from build123d import *

# Parameters (mm, degrees)
SKETCH4_R           = 59
BOSS_EXTRUDE3_DEPTH = 2
SKETCH5_R           = 1.375
BOSS_EXTRUDE5_DEPTH = 7
SKETCH8_R           = 2.375
BOSS_EXTRUDE6_DEPTH = 2
BOSS_EXTRUDE7_DEPTH = 18
SKETCH10_R          = 7.5
CUT_EXTRUDE1_DEPTH  = 18
SKETCH12_R          = 57.5
CUT_EXTRUDE2_DEPTH  = 5
CUT_EXTRUDE3_DEPTH  = 5.5
SKETCH15_R          = 89.714021058
SKETCH15_R_2        = 57
CUT_EXTRUDE4_DEPTH  = 22
SKETCH16_R          = 62.462022857
CUT_EXTRUDE8_DEPTH  = 52
CUT_EXTRUDE9_DEPTH  = 52
SKETCH18_R          = 80.62246508
SKETCH18_R_2        = 55
CUT_EXTRUDE10_DEPTH = 10
SKETCH19_R          = 55
BOSS_EXTRUDE8_DEPTH = 2
SKETCH20_R          = 6.25
CUT_EXTRUDE11_DEPTH = 2
SKETCH21_W          = 10
SKETCH21_H          = 50
CUT_EXTRUDE12_DEPTH = 3
SKETCH22_R          = 40.394642533
CUT_EXTRUDE13_DEPTH = 10


with BuildPart() as part:
    # Sketch4 → Boss-Extrude3 (new body)
    with BuildSketch(Plane.XY):
        Circle(SKETCH4_R)
    extrude(amount=BOSS_EXTRUDE3_DEPTH)

    # Sketch5 → Boss-Extrude5 (add)
    with BuildSketch(Plane.XY.offset(2)):
        with Locations((-22.5, 27.5)):
            Circle(SKETCH5_R)
        with Locations((22.5, 27.5)):
            Circle(SKETCH5_R)
        with Locations((22.5, -27.5)):
            Circle(SKETCH5_R)
        with Locations((-22.5, -27.5)):
            Circle(SKETCH5_R)
    extrude(amount=BOSS_EXTRUDE5_DEPTH)

    # Sketch8 → Boss-Extrude6 (add)
    with BuildSketch(Plane.XY.offset(2)):
        with Locations((-22.5, 27.5)):
            Circle(SKETCH8_R)
        with Locations((22.5, 27.5)):
            Circle(SKETCH8_R)
        with Locations((-22.5, -27.5)):
            Circle(SKETCH8_R)
        with Locations((22.5, -27.5)):
            Circle(SKETCH8_R)
    extrude(amount=BOSS_EXTRUDE6_DEPTH)

    # Sketch9 → Boss-Extrude7 (add)
    with BuildSketch(Plane.XY.offset(2)):
        with BuildLine():
            ThreePointArc((-4.745762712, 55.798546005), (0, 56), (4.745762712, 55.798546005))
            Line((4.745762712, 55.798546005), (5, 58.787753827))
            ThreePointArc((5, 58.787753827), (0, 59), (-5, 58.787753827))
            Line((-5, 58.787753827), (-4.745762712, 55.798546005))
        make_face()
        with BuildLine():
            Line((-55.798546005, 4.745762712), (-58.787753827, 5))
            ThreePointArc((-58.787753827, 5), (-59, 0), (-58.787753827, -5))
            Line((-58.787753827, -5), (-55.798546005, -4.745762712))
            ThreePointArc((-55.798546005, -4.745762712), (-56, 0), (-55.798546005, 4.745762712))
        make_face()
        with BuildLine():
            ThreePointArc((58.787753827, -5), (59, 0), (58.787753827, 5))
            Line((58.787753827, 5), (55.798546005, 4.745762712))
            ThreePointArc((55.798546005, 4.745762712), (56, 0), (55.798546005, -4.745762712))
            Line((55.798546005, -4.745762712), (58.787753827, -5))
        make_face()
        with BuildLine():
            ThreePointArc((-4.745762712, -55.798546005), (0, -56), (4.745762712, -55.798546005))
            Line((4.745762712, -55.798546005), (5, -58.787753827))
            ThreePointArc((5, -58.787753827), (0, -59), (-5, -58.787753827))
            Line((-5, -58.787753827), (-4.745762712, -55.798546005))
        make_face()
    extrude(amount=BOSS_EXTRUDE7_DEPTH)

    # Sketch10 → Cut-Extrude1 (cut)
    with BuildSketch(Plane.XY.offset(2)):
        with Locations((-40, 0)):
            Circle(SKETCH10_R)
    extrude(amount=-CUT_EXTRUDE1_DEPTH, mode=Mode.SUBTRACT)

    # Sketch12 → Cut-Extrude2 (cut)
    with BuildSketch(Plane.XY.offset(20)):
        Circle(SKETCH12_R)
    extrude(amount=-CUT_EXTRUDE2_DEPTH, mode=Mode.SUBTRACT)

    # Sketch13 → Cut-Extrude3 (cut)
    with BuildSketch(Plane(origin=(0, 0, 0), x_dir=(-1, 0, 0), z_dir=(0, 0, -1))):
        with BuildLine():
            Line((-57.243329786, 4.868644068), (-58.787753827, 5))
            ThreePointArc((-58.787753827, 5), (-59, 0), (-58.787753827, -5))
            Line((-58.787753827, -5), (-57.243329786, -4.868644068))
            ThreePointArc((-57.243329786, -4.868644068), (-57.45, 0), (-57.243329786, 4.868644068))
        make_face()
        with BuildLine():
            ThreePointArc((5, 58.787753827), (0, 59), (-5, 58.787753827))
            Line((-5, 58.787753827), (-4.868644068, 57.243329786))
            ThreePointArc((-4.868644068, 57.243329786), (0, 57.45), (4.868644068, 57.243329786))
            Line((4.868644068, 57.243329786), (5, 58.787753827))
        make_face()
        with BuildLine():
            Line((-4.868644068, -57.243329786), (-5, -58.787753827))
            ThreePointArc((-5, -58.787753827), (0, -59), (5, -58.787753827))
            Line((5, -58.787753827), (4.868644068, -57.243329786))
            ThreePointArc((4.868644068, -57.243329786), (0, -57.45), (-4.868644068, -57.243329786))
        make_face()
        with BuildLine():
            ThreePointArc((58.787753827, -5), (59, 0), (58.787753827, 5))
            Line((58.787753827, 5), (57.243329786, 4.868644068))
            ThreePointArc((57.243329786, 4.868644068), (57.45, 0), (57.243329786, -4.868644068))
            Line((57.243329786, -4.868644068), (58.787753827, -5))
        make_face()
    extrude(amount=-CUT_EXTRUDE3_DEPTH, mode=Mode.SUBTRACT)

    # Sketch15 → Cut-Extrude4 (cut)
    with BuildSketch(Plane(origin=(0, 0, 0), x_dir=(-1, 0, 0), z_dir=(0, 0, -1))):
        Circle(SKETCH15_R)
        Circle(SKETCH15_R_2, mode=Mode.SUBTRACT)
    extrude(amount=-CUT_EXTRUDE4_DEPTH, mode=Mode.SUBTRACT)

    # Sketch16 → Cut-Extrude8 (cut)
    with BuildSketch(Plane.XY.offset(2)):
        Circle(SKETCH16_R)
        with BuildLine():
            Line((55.798546005, 4.745762712), (56.794948612, 4.830508475))
            ThreePointArc((56.794948612, 4.830508475), (40.305086528, 40.305086528), (4.830508475, 56.794948612))
            Line((4.830508475, 56.794948612), (4.745762712, 55.798546005))
            ThreePointArc((4.745762712, 55.798546005), (0, 56), (-4.745762712, 55.798546005))
            Line((-4.745762712, 55.798546005), (-4.830508475, 56.794948612))
            ThreePointArc((-4.830508475, 56.794948612), (-40.305086528, 40.305086528), (-56.794948612, 4.830508475))
            Line((-56.794948612, 4.830508475), (-55.798546005, 4.745762712))
            ThreePointArc((-55.798546005, 4.745762712), (-56, 0), (-55.798546005, -4.745762712))
            Line((-55.798546005, -4.745762712), (-56.794948612, -4.830508475))
            ThreePointArc((-56.794948612, -4.830508475), (-40.305086528, -40.305086528), (-4.830508475, -56.794948612))
            Line((-4.830508475, -56.794948612), (-4.745762712, -55.798546005))
            ThreePointArc((-4.745762712, -55.798546005), (0, -56), (4.745762712, -55.798546005))
            Line((4.745762712, -55.798546005), (4.830508475, -56.794948612))
            ThreePointArc((4.830508475, -56.794948612), (40.305086528, -40.305086528), (56.794948612, -4.830508475))
            Line((56.794948612, -4.830508475), (55.798546005, -4.745762712))
            ThreePointArc((55.798546005, -4.745762712), (56, 0), (55.798546005, 4.745762712))
        make_face(mode=Mode.SUBTRACT)
    extrude(amount=CUT_EXTRUDE8_DEPTH, mode=Mode.SUBTRACT)

    # Sketch17 → Cut-Extrude9 (cut)
    with BuildSketch(Plane.XY.offset(2)):
        with BuildLine():
            Line((-5, 57), (5, 57))
            Line((5, 57), (4.806106124, 54.789609817))
            ThreePointArc((4.806106124, 54.789609817), (0, 55), (-4.806106124, 54.789609817))
            Line((-4.806106124, 54.789609817), (-5, 57))
        make_face()
        with BuildLine():
            Line((54.789609817, 4.806106124), (57, 5))
            Line((57, 5), (57, -5))
            Line((57, -5), (54.789609817, -4.806106124))
            ThreePointArc((54.789609817, -4.806106124), (55, 0), (54.789609817, 4.806106124))
        make_face()
        with BuildLine():
            Line((4.806106124, -54.789609817), (5, -57))
            Line((5, -57), (-5, -57))
            Line((-5, -57), (-4.806106124, -54.789609817))
            ThreePointArc((-4.806106124, -54.789609817), (0, -55), (4.806106124, -54.789609817))
        make_face()
        with BuildLine():
            Line((-54.789609817, -4.806106124), (-57, -5))
            Line((-57, -5), (-57, 5))
            Line((-57, 5), (-54.789609817, 4.806106124))
            ThreePointArc((-54.789609817, 4.806106124), (-55, 0), (-54.789609817, -4.806106124))
        make_face()
    extrude(amount=-CUT_EXTRUDE9_DEPTH, mode=Mode.SUBTRACT)

    # Sketch18 → Cut-Extrude10 (cut)
    with BuildSketch(Plane.XY.offset(2)):
        Circle(SKETCH18_R)
        Circle(SKETCH18_R_2, mode=Mode.SUBTRACT)
    extrude(amount=-CUT_EXTRUDE10_DEPTH, mode=Mode.SUBTRACT)

    # Sketch19 → Boss-Extrude8 (add)
    with BuildSketch(Plane.XY.offset(2)):
        Circle(SKETCH19_R)
    extrude(amount=-BOSS_EXTRUDE8_DEPTH)

    # Sketch20 → Cut-Extrude11 (cut)
    with BuildSketch(Plane.XY.offset(2)):
        with Locations((0, 44.5)):
            Circle(SKETCH20_R)
        with Locations((44.5, 0)):
            Circle(SKETCH20_R)
        with Locations((0, -44.5)):
            Circle(SKETCH20_R)
        with Locations((-44.5, 0)):
            Circle(SKETCH20_R)
    extrude(amount=-CUT_EXTRUDE11_DEPTH, mode=Mode.SUBTRACT)

    # Sketch21 → Cut-Extrude12 (cut)
    with BuildSketch(Plane.XY.offset(2)):
        with Locations((30, 0)):
            Rectangle(SKETCH21_W, SKETCH21_H)
        with Locations((-30, 0)):
            Rectangle(SKETCH21_W, SKETCH21_H)
    extrude(amount=-CUT_EXTRUDE12_DEPTH, mode=Mode.SUBTRACT)

    # Sketch22 → Cut-Extrude13 (cut)
    with BuildSketch(Plane.XY.offset(2)):
        Circle(SKETCH22_R)
    extrude(amount=CUT_EXTRUDE13_DEPTH, mode=Mode.SUBTRACT)


solid = part.part
Work out the finished part from the listing and answer in its coordinate system (mm). Round coordinates to 2 decimals unless told otherwise and drop trailing zeros. Order: outer loops, then holes, each group sorted by start corner. A loop starts at its lowest first (then second) coordinate and runs counter-clockwise, first axis right, second up. Notation, with made-up numbers: M 38.25,-21 L 86.25,-21 A9 ccw 86.25,-12 Z; hole C -29.5,81 d5. An arc over 180 degrees is marked long. One line per item, written item: value.
Q1. Determine the mould class of faces 1 (the face through (-1, 1, 2)), 2 (the face through (-0.8, 50.7, 1)) for opening direction Y: released by +Y, released by -Y, zero draft, split by the parting line, or undercut.
Derived:
face 1: zero draft
face 2: undercut
Q2. Find section D-D on x = -42.5. Write down the section's boundary in (y, z).
Derived:
outline: M -34.91,0 L -5.92,0 L -5.92,2 L -34.91,2 Z; M 5.92,0 L 34.91,0 L 34.91,2 L 5.92,2 Z
Q3. Find section B-B on z = 1.2. Write down the section's boundary in (x, y).
Derived:
outline: C 0,0 d110; hole C -44.5,0 d12.5; hole M -35,-25 L -25,-25 L -25,25 L -35,25 Z; hole C 0,-44.5 d12.5; hole C 0,44.5 d12.5; hole M 25,-25 L 35,-25 L 35,25 L 25,25 Z; hole C 44.5,0 d12.5
Q4. Straight lines are drawn through the part: line 1 (Y direction, x = 0, z = 0.75); line 2 (Y direction, x = 4.5, z = 1.65); line 3 (X direction, y = 2.5, z = 1.8). For each, find the intervals that lie inside material, in ascending order.
Derived:
line 1: -55 to -50.75, -38.25 to 38.25, 50.75 to 55
line 2: -54.82 to -48.84, -40.16 to 40.16, 48.84 to 54.82
line 3: -54.94 to -50.23, -38.77 to -35, -25 to 25, 35 to 38.77, 50.23 to 54.94
Q5. Find section C-C on x = 0. Write down the section's boundary in (y, z), then the cut area to 3 significant figures.
Derived:
outline: M -55,0 L -50.75,0 L -50.75,2 L -55,2 Z; M -38.25,0 L 38.25,0 L 38.25,2 L -38.25,2 Z; M 50.75,0 L 55,0 L 55,2 L 50.75,2 Z
area: 170 mm²
Q6. Flat-ended cylindrical pins translate along their axes: pin 1 (1 mm diameter, centred on x = 29, z = 0.5, fed in from -Y); pin 2 (1 mm diameter, centred on y = -9.5, z = 1.5, fed in from +X); pin 3 (0.6 mm diameter, centred on x = -31, z = 1.5, fed in from +Y). Find the tip coordinate at first contact, or state that the pin passes through.
Derived:
pin 1: y = -47.04
pin 2: x = 54.26
pin 3: y = 45.63
Q7. Find section A-A on y = 0. Write down the section's boundary in (x, z), then the cut area to 3 significant figures.
Derived:
outline: M -55,0 L -50.75,0 L -50.75,2 L -55,2 Z; M -38.25,0 L -35,0 L -35,2 L -38.25,2 Z; M -25,0 L 25,0 L 25,2 L -25,2 Z; M 35,0 L 38.25,0 L 38.25,2 L 35,2 Z; M 50.75,0 L 55,0 L 55,2 L 50.75,2 Z
area: 130 mm²
